Geometry: final body of the model. Coordinates: model frame, mm. Round coordinates to 2 decimals unless told otherwise and drop trailing zeros. Write each loop counter-clockwise with the first axis right and the second up, starting at its lowest first coordinate (ties: lowest second). Pieces come first, ordered by that corner, then holes.
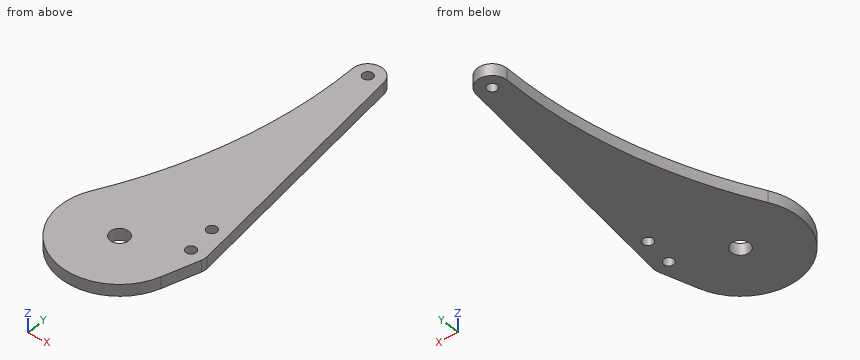
Autodesk Inventor part; units mm, degrees
ref_plane "YZ Plane" through (0, 0, 0) normal (1, 0, 0) x (0, 1, 0)
ref_plane "XZ Plane" through (0, 0, 0) normal (0, 1, 0) x (-1, 0, 0)
ref_plane "XY Plane" through (0, 0, 0) normal (0, 0, 1) x (1, 0, 0)
sketch "Sketch1" plane through (0, 0, 0) normal (0, 0, 1) x (1, 0, 0)
  circle A0 centre (1.835, -47.1215) radius 2.1844
  circle A1 centre (12.7, 69.85) radius 2.1844
  arc A2 (19.0097, 70.5645) -> (6.3511, 69.7333) centre (12.7, 69.85) ccw
  arc A3 (-20.2372, -34.5525) -> (25.9922, -54.9693) centre (1.835, -47.1215) ccw
  line L0 (25.9922, -54.9693) -> (30.9301, -39.7696)
  line L1 (31.2005, -37.0931) -> (19.0097, 70.5645)
  arc A4 (-20.2372, -34.5525) -> (6.3511, 69.7333) centre (-196.8146, 65.9992) ccw
  arc A5 (30.9301, -39.7696) -> (31.2005, -37.0931) centre (24.8908, -37.8076) ccw
  line L2 (5.0608, -43.8957) -> (-1.3908, -43.8957)
  line L3 (-1.3908, -43.8957) -> (-1.3908, -50.3473)
  line L4 (-1.3908, -50.3473) -> (5.0608, -50.3473)
  line L5 (5.0608, -50.3473) -> (5.0608, -43.8957)
  line L6 (5.0608, -43.8957) -> (-1.3908, -50.3473) construction
  line L7 (-1.3908, -43.8957) -> (5.0608, -50.3473) construction
  circle A6 centre (1.835, -47.1215) radius 3.937
  circle A7 centre (24.8908, -37.8076) radius 2.1844
  circle A8 centre (23.4618, -25.1883) radius 2.1844
  line L8 (24.8908, -37.8076) -> (23.4618, -25.1883)
  line L9 (1.835, -47.1215) -> (12.7, 69.85)
  point P0 (0, 0)
  dimension "d0" = 12.7
  dimension "d2" = 50.8
  dimension "d3" = 203.2
  dimension "d4" = 6.35
  dimension "d7" = 6.4516
  dimension "d8" = 6.4516
  dimension "d10" = 7.874
  dimension "d11" = 4.3688
  dimension "d12" = 4.3688
  dimension "d14" = 12.7
  dimension "d15" = 117.475
extrude "Extrusion1" add sketch "Sketch1" along normal blind 5.08 contours L2 L5 A6 | A6 L3 L2 | L5 L4 A6 | A6 L4 L3 | L1 A5 L0 A3 A4 A2
properties part number "intakeSide"
1) Line query: probe 1 along Y at (x, z) = (12.7, 3.05); probe 2 along Y at (x, z) = (12, 1.15); probe 3 along Y at (x, z) = (16, 1.65). Output: solid intervals per line, ascending.
2) Section A-A on x = 12.7. Output: boundary loops of the cut face in (y, z).
3) First-contact query: P1, Ø2, axis at x = -1, z = 1, coming from the -Y side; P2, Ø3.5, axis at x = 24.89, y = -37.81, coming from the +Z side; P3, Ø2, axis at x = 9.5, z = 1.5, coming from the -Y side; P4, Ø3, axis at y = -19, z = 2.5, coming from the -X side. Flat tips, straight axial feed; report the tip coordinate or a pass-through.
4) Section C-C on x = -4. Output: boundary loops of the cut face in (y, z).
5) Section B-B on y = -7. Output: boundary loops of the cut face in (x, z), plus the area to 3 significant figures.
Filled in:
1. probe 1: y = -70.08 to 67.67, 72.03 to 76.2
1. probe 2: y = -70.4 to 67.78, 71.92 to 76.16
1. probe 3: y = -68.2 to 75.28
2. outline: (-70.08, 0) - (67.67, 0) - (67.67, 5.08) - (-70.08, 5.08) - close; (72.03, 0) - (76.2, 0) - (76.2, 5.08) - (72.03, 5.08) - close
3. P1: stops at y = -72.46
3. P2: passes through
3. P3: stops at y = -71.63
3. P4: stops at x = -12.94
4. outline: (-71.84, 0) - (1.87, 0) - (1.87, 5.08) - (-71.84, 5.08) - close
5. outline: (-7.18, 0) - (27.79, 0) - (27.79, 5.08) - (-7.18, 5.08) - close
5. area: 178 mm2
